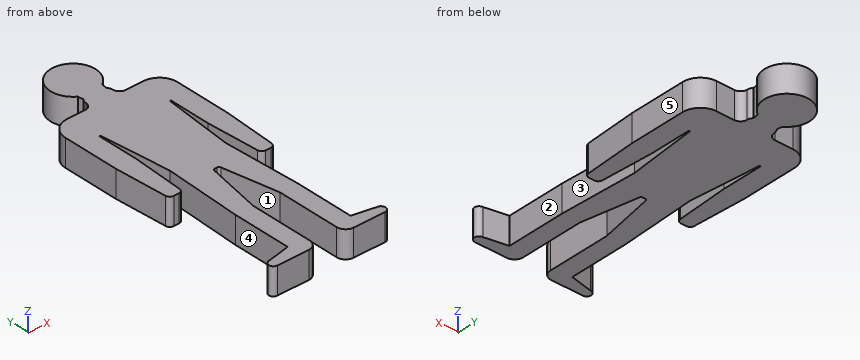
from build123d import *

# Parameters (mm, degrees)
SKETCH1_R            = 127
SKETCH1_W            = 76.2
SKETCH1_H            = 660.4
SKETCH1_W_2          = 101.6
SKETCH1_H_2          = 762
SKETCH1_W_3          = 228.6
SKETCH1_H_3          = 50.8
SKETCH1_W_4          = 152.4
SKETCH1_H_4          = 76.2
BOSS_EXTRUDE1_DEPTH  = 152.4
SKETCH2_W            = 406.4
SKETCH2_H            = 50.8
BOSS_EXTRUDE2_DEPTH  = 152.4
BOSS_EXTRUDE3_DEPTH  = 152.4
BOSS_EXTRUDE4_DEPTH  = 152.4
BOSS_EXTRUDE5_DEPTH  = 152.4
CUT_EXTRUDE1_DEPTH   = 152.4
SKETCH7_W            = 279.4
SKETCH7_H            = 114.872803244
BOSS_EXTRUDE6_DEPTH  = 152.4
BOSS_EXTRUDE7_DEPTH  = 152.4
SKETCH9_W            = 38.1
SKETCH9_H            = 736.6
BOSS_EXTRUDE8_DEPTH  = 152.4
FILLET2_R            = 101.6
CUT_EXTRUDE2_DEPTH   = 152.4
FILLET3_R            = 50.8
FILLET5_START        = -1
FILLET5_DEPTH        = 154
FILLET5_2_DEPTH      = 152.4
FILLET6_R            = 12.7
FILLET7_R            = 25.4
FILLET8_R            = 3.175
BOSS_EXTRUDE9_DEPTH  = 152.4
BOSS_EXTRUDE10_DEPTH = 152.4


with BuildPart() as part:
    # Sketch1 → Boss-Extrude1 (new body)
    with BuildSketch(Plane.XY):
        with Locations(Location((76.2, 1625.6, 0), (0, 0, 180))):
            Circle(SKETCH1_R)
        Polygon((-101.6, 812.8), (0, 812.8), (152.4, 812.8), (254, 812.8), (254, 1346.2), (254, 1422.4), (152.4, 1422.4), (0, 1422.4), (-101.6, 1422.4), (-101.6, 1346.2), align=None)
        Polygon((-127, 1346.2), (-101.6, 1346.2), (-101.6, 1422.4), (-203.2, 1422.4), (-203.2, 1346.2), align=None)
        with Locations((-165.1, 1016)):
            Rectangle(SKETCH1_W, SKETCH1_H)
        Polygon((254, 1422.4), (254, 1346.2), (279.4, 1346.2), (355.6, 1346.2), (355.6, 1422.4), align=None)
        with Locations((317.5, 1016)):
            Rectangle(SKETCH1_W, SKETCH1_H)
        with Locations((203.2, 431.8)):
            Rectangle(SKETCH1_W_2, SKETCH1_H_2)
        with Locations((-50.8, 431.8)):
            Rectangle(SKETCH1_W_2, SKETCH1_H_2)
        with Locations((-114.3, 25.4)):
            Rectangle(SKETCH1_W_3, SKETCH1_H_3)
        Polygon((254, 50.8), (152.4, 50.8), (152.4, 0), (381, 0), (381, 50.8), align=None)
        with BuildLine():
            ThreePointArc((381, 50.8), (406.4, 25.4), (381, 0))
            Line((381, 0), (381, 50.8))
        make_face()
        with BuildLine():
            ThreePointArc((-228.6, 0), (-254, 25.4), (-228.6, 50.8))
            Line((-228.6, 50.8), (-228.6, 0))
        make_face()
        with Locations((76.2, 1460.5)):
            Rectangle(SKETCH1_W_4, SKETCH1_H_4)
    extrude(amount=BOSS_EXTRUDE1_DEPTH)

    # Sketch2 → Boss-Extrude2 (add)
    with BuildSketch(Plane.XY.offset(152.4)):
        with Locations((76.2, 1320.8)):
            Rectangle(SKETCH2_W, SKETCH2_H)
    extrude(amount=-BOSS_EXTRUDE2_DEPTH)

    # Sketch3 → Boss-Extrude3 (add)
    with BuildSketch(Plane.XY.offset(152.4)):
        Polygon((76.2, 812.8), (0, 406.4), (0, 812.8), align=None)
    extrude(amount=-BOSS_EXTRUDE3_DEPTH)

    # Sketch4 → Boss-Extrude4 (add)
    with BuildSketch(Plane.XY.offset(152.4)):
        Polygon((76.2, 812.8), (152.4, 812.8), (152.4, 406.4), align=None)
    extrude(amount=-BOSS_EXTRUDE4_DEPTH)

    # Sketch5 → Boss-Extrude5 (add)
    with BuildSketch(Plane.XY.offset(152.4)):
        Polygon((-228.6, 50.8), (-101.6, 76.2), (-101.6, 50.8), align=None)
        Polygon((254, 76.2), (254, 50.8), (381, 50.8), align=None)
    extrude(amount=-BOSS_EXTRUDE5_DEPTH)

    # Sketch6 → Cut-Extrude1 (cut)
    with BuildSketch(Plane.XY.offset(152.4)):
        Polygon((-101.6, 406.4), (-81.750104461, 840.402248986), (-101.6, 1295.4), align=None)
        Polygon((254, 406.4), (234.150104461, 840.402248986), (254, 1295.4), align=None)
    extrude(amount=-CUT_EXTRUDE1_DEPTH, mode=Mode.SUBTRACT)

    # Sketch7 → Boss-Extrude6 (add)
    with BuildSketch(Plane.XY.offset(152.4)):
        with Locations((57.949895539, 782.965847364)):
            Rectangle(SKETCH7_W, SKETCH7_H)
    extrude(amount=-BOSS_EXTRUDE6_DEPTH)

    # Sketch8 → Boss-Extrude7 (add)
    with BuildSketch(Plane.XY.offset(152.4)):
        Polygon((-81.750104461, 840.402248986), (-127, 1295.4), (-61.647363893, 1295.4), align=None)
        Polygon((214.047363893, 1295.4), (234.150104461, 840.402248986), (279.4, 1295.4), align=None)
    extrude(amount=-BOSS_EXTRUDE7_DEPTH)

    # Sketch9 → Boss-Extrude8 (add)
    with BuildSketch(Plane.XY.offset(152.4)):
        with Locations((-222.25, 1054.1)):
            Rectangle(SKETCH9_W, SKETCH9_H)
        with Locations((374.65, 1054.1)):
            Rectangle(SKETCH9_W, SKETCH9_H)
    extrude(amount=-BOSS_EXTRUDE8_DEPTH)

    # Fillet2
    fillet2_edges = [part.edges().sort_by_distance(p)[0] for p in [
        (-241.3, 1422.4, 76.2),
        (393.7, 1422.4, 76.2),
    ]]
    fillet(fillet2_edges, radius=FILLET2_R)

    # Sketch10 → Cut-Extrude2 (cut)
    with BuildSketch(Plane.XY.offset(152.4)):
        Polygon((-241.3, 1003.3), (-222.469288436, 685.8), (-241.3, 685.8), align=None)
        Polygon((-145.830711564, 685.8), (-127, 685.8), (-127, 1003.3), align=None)
        Polygon((279.4, 1003.3), (298.230711564, 685.8), (279.4, 685.8), align=None)
        Polygon((374.869288436, 685.8), (393.7, 685.8), (393.7, 1003.3), align=None)
    extrude(amount=-CUT_EXTRUDE2_DEPTH, mode=Mode.SUBTRACT)

    # Fillet3
    fillet3_edges = [part.edges().sort_by_distance(p)[0] for p in [
        (152.4, 0, 76.2),
        (0, 0, 76.2),
    ]]
    fillet(fillet3_edges, radius=FILLET3_R)

    # Fillet5: read off the stored shape, not the designer's step
    # Fillet5 outline → Fillet5 (cut)
    with BuildSketch(Plane.XY.offset(FILLET5_START)):
        with BuildLine():
            ThreePointArc((0, 1460.5), (11.159231637, 1487.440768363), (38.1, 1498.6))
            Line((38.1, 1498.6), (0, 1498.6))
            Line((0, 1498.6), (0, 1460.5))
        make_face()
        with BuildLine():
            ThreePointArc((114.3, 1498.6), (141.240768363, 1487.440768363), (152.4, 1460.5))
            Line((152.4, 1460.5), (152.4, 1498.6))
            Line((152.4, 1498.6), (114.3, 1498.6))
        make_face()
    extrude(amount=FILLET5_DEPTH, mode=Mode.SUBTRACT)

    # Fillet5 2 outline → Fillet5 2 (add)
    with BuildSketch(Plane.XY):
        with BuildLine():
            Line((152.4, 1422.4), (190.5, 1422.4))
            ThreePointArc((190.5, 1422.4), (163.559231637, 1433.559231637), (152.4, 1460.5))
            Line((152.4, 1460.5), (152.4, 1422.4))
        make_face()
        with BuildLine():
            Line((0, 1422.4), (0, 1460.5))
            ThreePointArc((0, 1460.5), (-11.159231637, 1433.559231637), (-38.1, 1422.4))
            Line((-38.1, 1422.4), (0, 1422.4))
        make_face()
    extrude(amount=FILLET5_2_DEPTH)

    # Fillet6
    fillet6_edges = [part.edges().sort_by_distance(p)[0] for p in [
        (92.563228923, 725.529445742, 76.2),
        (59.836771077, 725.529445742, 76.2),
    ]]
    fillet(fillet6_edges, radius=FILLET6_R)

    # Fillet7
    fillet7_edges = [part.edges().sort_by_distance(p)[0] for p in [
        (-222.469288436, 685.8, 76.2),
        (-145.830711564, 685.8, 76.2),
        (298.230711564, 685.8, 76.2),
        (374.869288436, 685.8, 76.2),
    ]]
    fillet(fillet7_edges, radius=FILLET7_R)

    # Fillet8
    fillet8_edges = [part.edges().sort_by_distance(p)[0] for p in [
        (279.4, 1295.4, 76.2),
        (-127, 1295.4, 76.2),
    ]]
    fillet(fillet8_edges, radius=FILLET8_R)

    # Sketch11 → Boss-Extrude9 (add)
    with BuildSketch(Plane.XY.offset(152.4)):
        Polygon((6.96991061, 1519.128432325), (11.159231637, 1487.440768363), (76.2, 1498.6), align=None)
    extrude(amount=-BOSS_EXTRUDE9_DEPTH)

    # Sketch12 → Boss-Extrude10 (add)
    with BuildSketch(Plane.XY.offset(152.4)):
        Polygon((145.43008939, 1519.128432325), (76.2, 1498.6), (141.240768363, 1487.440768363), align=None)
    extrude(amount=-BOSS_EXTRUDE10_DEPTH)


solid = part.part
The model under review builds one solid part; all positions refer to its coordinate system, in mm. Face numbers are marked on the shaded views. A direction names the side the tool comes from. Coordinates: 2 decimals unless noted, no trailing zeros. Order: outer loops, then holes, each group sorted by start corner. A loop starts at its lowest first (then second) coordinate and runs counter-clockwise, first axis right, second up. Notation, with made-up numbers: (50, 68.25) -> (61, 68.25) arc R26 ccw to (61, 100.25) -> close; hole circle Ø3 at (6.5, 13). An arc over 180 degrees is marked (long way). Answer in a Markdown table with one row per item.
(1) Consider section B-B (y = 437). Write out the cut boundary in (x, z), plus the area to 3 significant figures.
Answers:
| item | result |
|---|---|
| outline | (-100.2, 0) -> (5.74, 0) -> (5.74, 152.4) -> (-100.2, 152.4) -> close; (146.66, 0) -> (252.6, 0) -> (252.6, 152.4) -> (146.66, 152.4) -> close |
| area | 32,300 mm² |
(2) Consider section D-D (y = 1625.6). Write out the cut boundary in (x, z), plus the area to 3 significant figures.
Answers:
| item | result |
|---|---|
| outline | (-50.8, 0) -> (203.2, 0) -> (203.2, 152.4) -> (-50.8, 152.4) -> close |
| area | 38,700 mm² |
(3) Consider section C-C (y = 25.4). Write out the cut boundary in (x, z), plus the area to 3 significant figures.
Answers:
| item | result |
|---|---|
| outline | (-254, 0) -> (-6.81, 0) -> (-6.81, 152.4) -> (-254, 152.4) -> close; (159.21, 0) -> (406.4, 0) -> (406.4, 152.4) -> (159.21, 152.4) -> close |
| area | 75,300 mm² |
(4) Consider section A-A (y = 937). Write out the cut boundary in (x, z), plus the area to 3 significant figures.
Answers:
| item | result |
|---|---|
| outline | (-237.37, 0) -> (-130.93, 0) -> (-130.93, 152.4) -> (-237.37, 152.4) -> close; (-91.36, 0) -> (243.76, 0) -> (243.76, 152.4) -> (-91.36, 152.4) -> close; (283.33, 0) -> (389.77, 0) -> (389.77, 152.4) -> (283.33, 152.4) -> close |
| area | 83,500 mm² |
(5) Wall thickness on line 1 along X through (y, z) = (142.5, 78); line 2 along X through (y, z) = (964, 95); line 3 along X through (y, z) = (763, 131): over which ranges is each line inside the solid? List them lowest first.
Answers:
| item | result |
|---|---|
| line 1 | -101.6 to 0, 152.4 to 254 |
| line 2 | -238.97 to -129.33, -94.04 to 246.44, 281.73 to 391.37 |
| line 3 | -227.05 to -141.25, -85.29 to 237.69, 293.65 to 379.45 |
(6) Insertion check: pin 1 (10 mm diameter, centred on y = 991.5, z = 81, fed in from -X); pin 2 (9.5 mm diameter, centred on x = 79, z = 78.5, fed in from -Y); pin 3 (5 mm diameter, centred on x = 1.5, z = 31.5, fed in from +Y). Each pin has a flat end and moves straight along its axis. Give the tip position at first contact, or say it passes through.
Answers:
| item | result |
|---|---|
| pin 1 | x = -240.9 |
| pin 2 | y = 725.41 |
| pin 3 | y = 1730.08 |
(7) Machinability: for the marked faces 1, 2, 3, 4 and 5, which of the approach directions +Z, -Z, +X, -X, +Y, -Y give a long, thin tool a straight path to every point of the face, cutting with its end or side? Answer none if there is none.
Answers:
| item | result |
|---|---|
| face 1 | +Z, -Z, -Y |
| face 2 | +Z, -Z, +X |
| face 3 | +Z, -Z |
| face 4 | +Z, -Z, -X |
| face 5 | +Z, -Z, +X, +Y |
